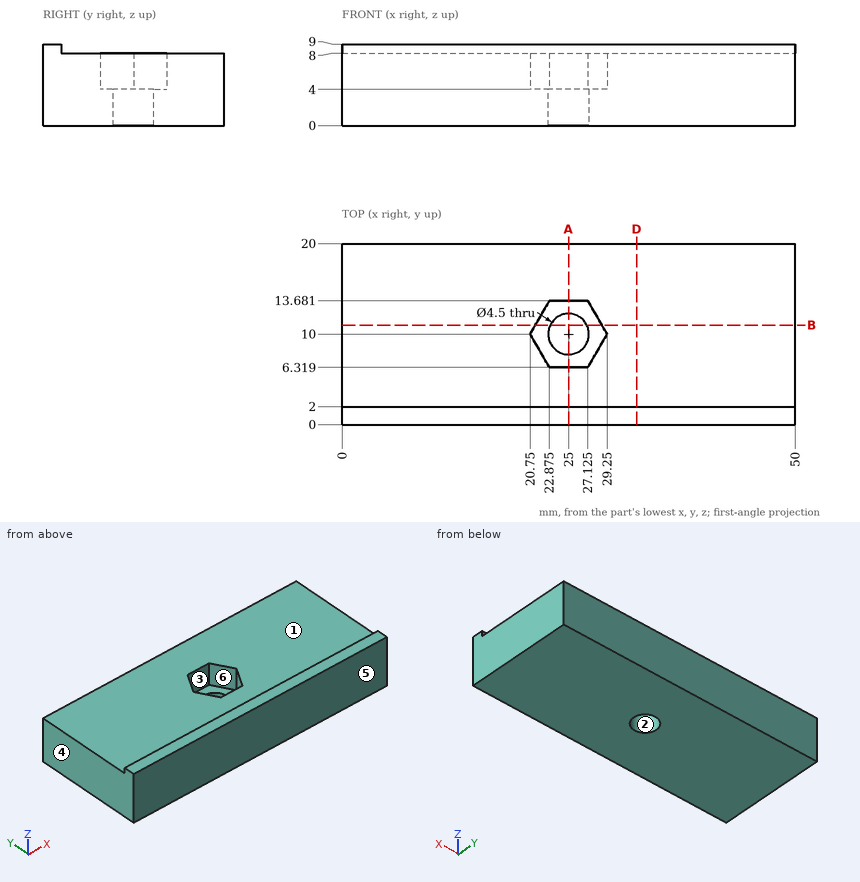
The drawing under review shows one solid part. Ordinate dimensions are in mm from its lowest x, y, z. A direction names the side the tool comes from. Round coordinates to 2 decimals unless told otherwise and drop trailing zeros. Write each loop counter-clockwise with the first axis right and the second up, starting at its lowest first coordinate (ties: lowest second). Pieces come first, ordered by that corner, then holes. Notation, with made-up numbers: (37, -11.75) -> (81, -11.75) arc R21 cw to (81, 6.25) -> close; hole circle Ø11 at (14, 14). An arc over 180 degrees is marked (long way). One line per question, with ' | ' between items. Start each with the question number.
(1) Tool access review of the marked faces 1, 2 and 3: name each direction out of +Z, -Z, +X, -X, +Y, -Y from which nothing blocks a thin tool from reaching the whole face with its end or side.
(2) For line 1 along Y through (x, z) = (25, 1.4); line 2 along Z through (x, y) = (26.5, 16.25); line 3 along Y through (x, z) = (25.5, 5.5), list the stretches that pass through material, from the lowest coordinate up. Write a range as from..to.
(3) Add section B-B, the plane y = 11. Write out the cut boundary in (x, z) (1 decimal).
(4) Mouldability with a two-part tool opening along Y and no side actions: class the marked faces 4, 5 and 6 as released by +Y, released by -Y, zero draft, split by the parting line, or undercut.
(5) Insertion check: P1, Ø2, axis at x = 43.5, y = 17.5, coming from the +Z side; P2, Ø2, axis at x = 26.5, y = 11.5, coming from the +Z side; P3, Ø2.5, axis at x = 25, y = 10, coming from the -Z side. Each pin has a flat end and moves straight along its axis. Give the tip position at first contact, or say it passes through.
(6) Add section D-D, the plane x = 32.5. Write out the cut boundary in (y, z).
(7) Add section A-A, the plane x = 25. Write out the cut boundary in (y, z).
Answer list:
1) face 1: +Z, +X, -X, +Y | face 2: +Z, -Z | face 3: +Z
2) line 1: 0..7.75, 12.25..20 | line 2: 0..8 | line 3: 0..6.32, 13.68..20
3) outline: (0, 0) -> (23, 0) -> (23, 4) -> (21.3, 4) -> (21.3, 8) -> (0, 8) -> close; (27, 0) -> (50, 0) -> (50, 8) -> (28.7, 8) -> (28.7, 4) -> (27, 4) -> close
4) face 4: zero draft | face 5: released by -Y | face 6: undercut
5) P1: z = 8 | P2: z = 4 | P3: through
6) outline: (0, 0) -> (20, 0) -> (20, 8) -> (2, 8) -> (2, 9) -> (0, 9) -> close
7) outline: (0, 0) -> (7.75, 0) -> (7.75, 4) -> (6.32, 4) -> (6.32, 8) -> (2, 8) -> (2, 9) -> (0, 9) -> close; (12.25, 0) -> (20, 0) -> (20, 8) -> (13.68, 8) -> (13.68, 4) -> (12.25, 4) -> close
